The listing builds one solid part. Answer for the finished solid, in the listing's coordinates (mm). Face numbers are marked on the shaded views. Round coordinates to 2 decimals unless told otherwise and drop trailing zeros. Write each loop counter-clockwise with the first axis right and the second up, starting at its lowest first coordinate (ties: lowest second). Pieces come first, ordered by that corner, then holes. Notation, with made-up numbers: M 9,8 L 17,8 A18 ccw 17,26 Z; hole C 60,87.5 d10. An arc over 180 degrees is marked long. Answer as CSV lines item,"result". Start each with the question number.
Autodesk Fusion 360 part; units mm, degrees
sketch "Sketch1" plane through (0, 0, 0) normal (0, 1, 0) x (1, 0, 0)
  line L0 (0, 0) -> (-140, 0)
  line L1 (-140, 0) -> (-140, 140)
  line L2 (-140, 140) -> (0, 140)
  line L3 (0, 140) -> (0, 0)
  dimension "d1" = 140
  dimension "d2" = 140
extrude "Extrude1" add sketch "Sketch1" along normal blind 2 makes body 1
sketch "Sketch2" plane through (0, 2, 0) normal (0, 1, 0) x (-1, 0, 0)
  line L0 (0, -140) -> (140, -140)
  line L1 (140, -140) -> (140, 0)
  line L2 (140, 0) -> (0, 0)
  line L3 (0, 0) -> (0, -140)
  line L4 (70, -140) -> (23, -140)
  line L5 (117, -140) -> (116, -140)
  line L6 (117, -140) -> (117.75, -140)
  line L7 (117.75, -140) -> (116.25, -140)
  line L8 (117.75, -140) -> (116.25, -140)
  line L9 (116.25, -140) -> (116.25, 0)
  line L10 (116.25, 0) -> (117.75, 0)
  line L11 (117.75, 0) -> (117.75, -140)
  dimension "d5" = 47
  dimension "d6" = 47
  dimension "d7" = 0.75
  dimension "d8" = 1.5
extrude "Extrude2" add sketch "Sketch2" along normal blind 2 contours L0 L2 L5 L6 L7 L8 L9 L10 L11 bodies 1
sketch "Sketch3" plane through (0, 2, 0) normal (0, 1, 0) x (-1, 0, 0)
  line L0 (116.25, -140) -> (116.25, 0)
  line L1 (116.25, 0) -> (0, 0)
  line L2 (0, 0) -> (0, -140)
  line L3 (0, -140) -> (116.25, -140)
  line L4 (0, -140) -> (22.25, -140)
  line L5 (22.25, -140) -> (20.75, -140)
  line L6 (20.75, -140) -> (20.75, 0)
  line L7 (20.75, 0) -> (22.25, 0)
  line L8 (22.25, 0) -> (22.25, -140)
  dimension "d11" = 22.25
  dimension "d12" = 1.5
extrude "Extrude3" add sketch "Sketch3" along normal blind 2 contours L1 L3 L4 L5 L6 L7 L8 bodies 1
sketch "Sketch4" plane through (0, 2, 0) normal (0, 1, 0) x (-1, 0, 0)
extrude "Extrude4" add 1 faces at (0, 0.6667, -93.3333) along direction (1, 0, 0) blind 10 on bodies 1 bodies 1
extrude "Extrude5" add 1 faces at (-140, 0.6667, -46.6667) along direction (-1, 0, 0) blind 10 on bodies 1 bodies 1
sketch "Sketch5" plane through (0, 2, 0) normal (0, 1, 0) x (-1, 0, 0)
  line L0 (20.75, -140) -> (20.75, 0)
  line L1 (20.75, 0) -> (-10, 0)
  line L2 (-10, 0) -> (-10, -140)
  line L3 (-10, -140) -> (20.75, -140)
  line L4 (0.75, -140) -> (-2.25, -140)
  line L5 (-2.25, -140) -> (-2.25, 0)
  line L6 (-2.25, 0) -> (0.75, 0)
  line L7 (0.75, 0) -> (0.75, -140)
  dimension "d19" = 20
  dimension "d20" = 3
  dimension "d21" = 140
extrude "Extrude6" add sketch "Sketch5" along normal blind 3 contours L1 L3 L4 L5 L6 L7 bodies 1
sketch "Sketch6" plane through (0, 2, 0) normal (0, 1, 0) x (-1, 0, 0)
  line L0 (117.75, 0) -> (117.75, -140)
  line L1 (117.75, -140) -> (150, -140)
  line L2 (150, -140) -> (150, 0)
  line L3 (150, 0) -> (117.75, 0)
  line L4 (137.75, -140) -> (140.75, -140)
  line L5 (140.75, -140) -> (140.75, 0)
  line L6 (140.75, 0) -> (137.75, 0)
  line L7 (137.75, 0) -> (137.75, -140)
  dimension "d24" = 20
  dimension "d25" = 3
  dimension "d26" = 140
extrude "Extrude7" add sketch "Sketch6" along normal blind 3 contours L1 L3 L4 L5 L6 L7 bodies 1
sketch "Sketch7" plane through (0, 5, 0) normal (0, 1, 0) x (-1, 0, 0)
sketch "Sketch8" plane through (0, 2, 0) normal (0, 1, 0) x (-1, 0, 0)
sketch "Sketch9" plane through (0, 5, 0) normal (0, 1, 0) x (-1, 0, 0)
sketch "Sketch10" plane through (0, 5, 0) normal (0, 1, 0) x (-1, 0, 0)
sketch "Sketch11" plane through (0, 2, 0) normal (0, 1, 0) x (-1, 0, 0)
  line L0 (22.25, -140) -> (116.25, -140)
  line L1 (116.25, -140) -> (116.25, 0)
  line L2 (116.25, 0) -> (22.25, 0)
  line L3 (23.25, 0) -> (21.75, 0)
  line L4 (21.75, 0) -> (21.75, -140)
  line L5 (21.75, -140) -> (23.25, -140)
  line L6 (23.25, -140) -> (23.25, 0)
  dimension "d29" = 1
  dimension "d30" = 1.5
extrude "Extrude8" cut 1 faces at (-21.75, 4, -93.3333) along direction (0, -1, 0) blind 2 on bodies 1 bodies 1
extrude "Extrude9" add sketch "Sketch11" along normal blind 2 contours L0 L2 L3 L4 L5 L6 bodies 1
extrude "Extrude10" cut 1 faces at (-116.75, 4, -93.3333) along direction (0, -1, 0) blind 2 on bodies 1 bodies 1
sketch "Sketch12" plane through (0, 2, 0) normal (0, 1, 0) x (-1, 0, 0)
  line L0 (23.25, 0) -> (23.25, -140)
  line L1 (23.25, -140) -> (137.75, -140)
  line L2 (137.75, -140) -> (137.75, 0)
  line L3 (137.75, 0) -> (23.25, 0)
  line L4 (23.25, -140) -> (115.25, -140)
  line L5 (115.25, -140) -> (116.75, -140)
  line L6 (116.75, -140) -> (116.75, 0)
  line L7 (116.75, 0) -> (115.25, 0)
  line L8 (115.25, 0) -> (115.25, -140)
  dimension "d37" = 92
  dimension "d38" = 1.5
extrude "Extrude11" add sketch "Sketch12" along normal blind 2 contours L1 L3 L5 L6 L7 L8 bodies 1
sketch "Sketch13" plane through (0, 2, 0) normal (0, 1, 0) x (-1, 0, 0)
copy_body "Body->Comp1" bodies 1 removing the originals makes body 2 in component "Component"
extrude "Extrude1'" add 1 faces at (-92.5833, 0.6667, 0) along direction (0, 0, 1) blind 75 on bodies 2 bodies 2 in component "Component"
component "Component" placed x (1, 0, 0) y (0, 1, 0) z (0, 0, 1) at (0, 0, 0)
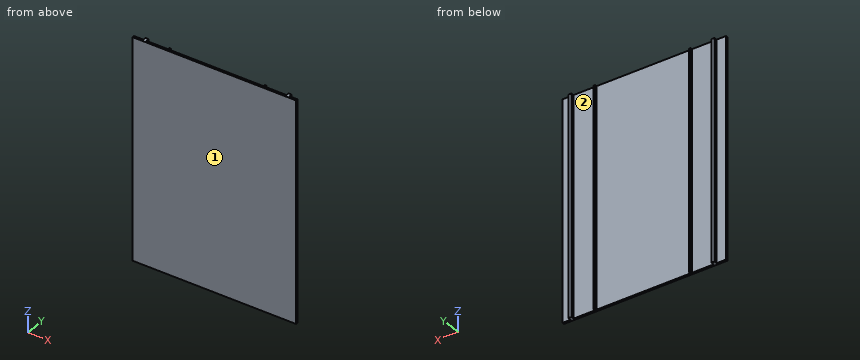
Q1. Straight lines are drawn through the part: L1, parallel to X at y = 2.95, z = -82.5; L2, parallel to X at y = 4.4, z = 27.5; L3, parallel to Y at x = 3.5, z = -109. For each, find the intervals that lie inside material, in ascending order.
Q2. Find section C-C (x = -29.5). Determine the outline of the cut face in (y, z), plus the area to 3 significant figures.
Q3. Each of these flat-tipped pins is pushed along its axis until it touches: P1, Ø17, axis at x = -132.5, z = -69.5, coming from the +Y side; P2, Ø0.9, axis at y = 3, z = -46, coming from the -X side; P3, Ø2, axis at x = -20.5, z = -12.5, coming from the +Y side; P4, Ø2, axis at y = 3.5, z = 14, coming from the +X side. Where does it stop, or does it pass through?
Q4. The mould has two halves that part along X. Classify the marked faces 1 and 2: +X half, -X half, draft (parallel to the pull), parting line (faces both ways), or undercut.
Q5. Find section A-A (y = 3.15). Determine the outline of the cut face in (x, z).
Q6. Find section B-B (z = -9). Determine the outline of the cut face in (x, y).
Reported:
1,L1,"x = -140.75 to -137.75, -116.75 to -115.25, -23.25 to -21.75, -0.75 to 2.25"
1,L2,"x = -140.75 to -137.75, -0.75 to 2.25"
1,L3,"y = 0 to 2"
2,outline,"M 0,-140 L 2,-140 L 2,75 L 0,75 Z"
2,area,"430 mm2"
3,P1,"stops at y = 5"
3,P2,"stops at x = -140.75"
3,P3,"stops at y = 2"
3,P4,"stops at x = 2.25"
4,face 1,"draft"
4,face 2,"undercut"
5,outline,"M -140.75,-140 L -137.75,-140 L -137.75,75 L -140.75,75 Z; M -116.75,-140 L -115.25,-140 L -115.25,75 L -116.75,75 Z; M -23.25,-140 L -21.75,-140 L -21.75,75 L -23.25,75 Z; M -0.75,-140 L 2.25,-140 L 2.25,75 L -0.75,75 Z"
6,outline,"M -150,0 L 10,0 L 10,2 L 2.25,2 L 2.25,5 L -0.75,5 L -0.75,2 L -21.75,2 L -21.75,4 L -23.25,4 L -23.25,2 L -115.25,2 L -115.25,4 L -116.75,4 L -116.75,2 L -137.75,2 L -137.75,5 L -140.75,5 L -140.75,2 L -150,2 Z"
